Model file for the job. Use its own axes, mm. A direction names the side the tool comes from. Coordinates: 2 decimals unless noted, no trailing zeros. Loops run counter-clockwise (first coordinate to the right, second up) from the corner with the lowest first, then second, coordinate; pieces in that order, holes last.
from build123d import *

# Parameters (mm, degrees)
Y_KSEKLIK_EKSTR_ZYON1_DEPTH = 10
IZIM3_W                     = 33
IZIM3_H                     = 33
KES_EKSTR_ZYON1_DEPTH       = 10
KES_EKSTR_ZYON1_DRAFT       = -40.36453657
IZIM7_OUTSIDE_W             = 57.326
IZIM7_OUTSIDE_H             = 24.326
KES_EKSTR_ZYON6_DEPTH       = 56
IZIM10_OUTSIDE_W            = 24.326
IZIM10_OUTSIDE_H            = 57.326
KES_EKSTR_ZYON8_DEPTH       = 28
Y_KSEKLIK_EKSTR_ZYON2_DEPTH = 39
IZIM12_R                    = 14.5
Y_KSEKLIK_EKSTR_ZYON3_DEPTH = 100
Y_KSEKLIK_EKSTR_ZYON4_DEPTH = 2


with BuildPart() as part:
    # Çizim2 → Yükseklik-Ekstrüzyon1 (new body)
    with BuildSketch(Plane.XY):
        Polygon((0, 16.5), (0, 21.5), (-21.5, 21.5), (-21.5, 0), (-16.5, 0), (-16.5, 16.5), align=None)
        Polygon((0, 8), (0, 16.5), (-16.5, 16.5), (-16.5, 0), (-8, 0), (-8, 8), align=None)
        Polygon((-21.5, -21.5), (0, -21.5), (0, -16.5), (-16.5, -16.5), (-16.5, 0), (-21.5, 0), align=None)
        Polygon((-16.5, -16.5), (0, -16.5), (0, -8), (-8, -8), (-8, 0), (-16.5, 0), align=None)
        Polygon((21.5, -21.5), (21.5, 0), (16.5, 0), (16.5, -16.5), (0, -16.5), (0, -21.5), align=None)
        Polygon((16.5, -16.5), (16.5, 0), (8, 0), (8, -8), (0, -8), (0, -16.5), align=None)
        Polygon((8, 0), (16.5, 0), (16.5, 16.5), (0, 16.5), (0, 8), (8, 8), align=None)
        Polygon((16.5, 0), (21.5, 0), (21.5, 21.5), (0, 21.5), (0, 16.5), (16.5, 16.5), align=None)
    extrude(amount=Y_KSEKLIK_EKSTR_ZYON1_DEPTH)


with BuildPart() as kes_ekstr_zyon1_tool:
    # Çizim3 → Kes-Ekstrüzyon1 (with draft: the straight prism first)
    with BuildSketch(Plane.XY.offset(10)):
        Rectangle(IZIM3_W, IZIM3_H)
    extrude(amount=-KES_EKSTR_ZYON1_DEPTH)
    # Kes-Ekstrüzyon1: the draft: its side faces are tilted about the plane it starts from
    kes_ekstr_zyon1_sides = [kes_ekstr_zyon1_tool.faces().sort_by_distance(p)[0] for p in [
        (-16.5, 0, 5),
        (0, -16.5, 5),
        (16.5, 0, 5),
        (0, 16.5, 5),
    ]]
    draft(kes_ekstr_zyon1_sides, Plane.XY.offset(10), KES_EKSTR_ZYON1_DRAFT)


with BuildPart() as part_1:
    add(part.part)

    # Kes-Ekstrüzyon1: cut by kes_ekstr_zyon1_tool
    add(kes_ekstr_zyon1_tool.part, mode=Mode.SUBTRACT)

    # Çizim7 outside → Kes-Ekstrüzyon6 (cut)
    with BuildSketch(Plane(origin=(0, 21.5, 0), x_dir=(1, 0, 0), z_dir=(0, 1, 0))):
        with Locations((0, -5)):
            Rectangle(IZIM7_OUTSIDE_W, IZIM7_OUTSIDE_H)
        Polygon((-21.5, -10), (21.5, -10), (13, 0), (-13, 0), align=None, mode=Mode.SUBTRACT)
    extrude(amount=-KES_EKSTR_ZYON6_DEPTH, mode=Mode.SUBTRACT)

    # Çizim10 outside → Kes-Ekstrüzyon8 (cut, symmetric)
    with BuildSketch(Plane(origin=(0, 0, 0), x_dir=(0, 0, -1), z_dir=(1, 0, 0))):
        with Locations((-5, 0)):
            Rectangle(IZIM10_OUTSIDE_W, IZIM10_OUTSIDE_H)
        Polygon((-10, 21.5), (-10, -21.5), (0, -13), (0, 13), align=None, mode=Mode.SUBTRACT)
    extrude(amount=KES_EKSTR_ZYON8_DEPTH, both=True, mode=Mode.SUBTRACT)

    # Çizim11 → Yükseklik-Ekstrüzyon2 (add)
    with BuildSketch(Plane(origin=(0, 0, 0), x_dir=(-1, 0, 0), z_dir=(0, 0, -1))):
        Polygon((-13, -13), (-32.5, -32.5), (32.5, -32.5), (32.5, 32.5), (13, 13), (13, -13), align=None)
        Polygon((-32.5, 32.5), (-32.5, -32.5), (-13, -13), (-13, 13), (13, 13), (32.5, 32.5), align=None)
        Polygon((-13, 13), (-13, -13), (-8.000000001, -8.000000001), (-8, 8), (8.000000001, 8.000000001), (13, 13), align=None)
        Polygon((-8, 8), (-8.000000001, -8.000000001), (8.000000001, 8.000000001), align=None)
        Polygon((8.000000001, 8.000000001), (-8.000000001, -8.000000001), (8.000000001, -8.000000001), align=None)
        Polygon((-8.000000001, -8.000000001), (-13, -13), (13, -13), (13, 13), (8.000000001, 8.000000001), (8.000000001, -8.000000001), align=None)
    extrude(amount=Y_KSEKLIK_EKSTR_ZYON2_DEPTH)

    # Çizim12 → Yükseklik-Ekstrüzyon3 (add)
    with BuildSketch(Plane.XZ.offset(32.5)):
        with Locations((0, -19.5)):
            Circle(IZIM12_R)
    extrude(amount=Y_KSEKLIK_EKSTR_ZYON3_DEPTH)

    # Çizim13 → Yükseklik-Ekstrüzyon4 (add)
    with BuildSketch(Plane.XZ.offset(132.5)):
        Polygon((-1, -31.880933569), (1, -31.880933569), (0, -33.652876783), align=None)
        Polygon((-3.663034054, -33.170629201), (-2.238495577, -31.717882533), (-4.17034723, -31.200244443), align=None)
        Polygon((-7.076438392, -31.756750831), (-5.324441381, -30.722202993), (-7.056492188, -29.722202993), align=None)
        Polygon((-10.007595147, -29.507595147), (-8.047535303, -28.961748865), (-9.461748865, -27.547535303), align=None)
        Polygon((-12.256750831, -26.576438392), (-10.222202993, -26.556492188), (-11.222202993, -24.824441381), align=None)
        Polygon((-13.670629201, -23.163034054), (-11.700244443, -23.67034723), (-12.217882533, -21.738495578), align=None)
        Polygon((-14.152876783, -19.5), (-12.380933569, -20.5), (-12.380933569, -18.5), align=None)
    extrude(amount=Y_KSEKLIK_EKSTR_ZYON4_DEPTH)


solid = part_1.part
Q1. Which spindle directions (+Z, -Z, +X, -X, +Y, -Y) get a long thin tool onto all of the face, cutting with end or side? Do faces 4 (the flat face through (17.31, 0.3, 5.07)), 5 (the flat face through (-13.254, -0.231, 6.181)), 6 (the flat face through (0.3, 17.19, 4.93)). Say none if no direction does.
Answers:
face 4: +X, +Y, -Y
face 5: +Z
face 6: +X, -X, +Y
Q2. Drill centre lines: line 1 (Z direction, x = -3, y = -49.5); line 2 (Y direction, x = -9.5, z = -22.5); line 3 (Y direction, x = 10, z = -8). Where is each one in solid material? Low to high.
Answers:
line 1: z = -33.69 to -5.31
line 2: y = -132.5 to 32.5
line 3: y = -32.5 to 32.5
Q3. Mould opens along Y. For faces 1 (the flat face through (0, 0, 0)), 2 (the flat face through (0, 0, -39)), 3 (the flat face through (0, 32.5, -19)) say: +Y half, -Y half, draft (parallel to the pull), parting line (faces both ways), or undercut.
Answers:
face 1: undercut
face 2: draft
face 3: +Y half
Q4. Slice it at B-B (z = -9). List the corners of the cut face in (x, y), and give its area (4 significant figures).
Answers:
outline: (-32.5, -32.5) - (-10, -32.5) - (-10, -132.5) - (10, -132.5) - (10, -32.5) - (32.5, -32.5) - (32.5, 32.5) - (-32.5, 32.5) - close
area: 6,225 mm2
Q5. Slice it at C-C (z = 4.5). List the corners of the cut face in (x, y) (3 decimals).
Answers:
outline: (-16.825, -16.825) - (16.825, -16.825) - (16.825, 16.825) - (-16.825, 16.825) - close; hole (-11.825, -11.825) - (11.825, -11.825) - (11.825, 11.825) - (-11.825, 11.825) - close
Q6. Flat gauge pins, fed straight in: P1, Ø4, axis at x = 3, z = -3, coming from the -Y side; P2, Ø1.5, axis at y = -96.5, z = -10.5, coming from the -X side; P3, Ø11.5, axis at x = -5, z = -16.5, coming from the -Y side. Where does each tip first touch, or does it go through?
Answers:
P1: stops at y = -32.5
P2: stops at x = -11.92
P3: stops at y = -132.5
Q7. Slice it at D-D (y = -72). List the corners of the cut face in (x, z), and give its area (3 significant figures).
Answers:
outline: circle Ø29 at (0, -19.5)
area: 661 mm2
Q8. Slice it at A-A (y = 20). List the corners of the cut face in (x, z), and give its area (3 significant figures).
Answers:
outline: (-32.5, -39) - (32.5, -39) - (32.5, 0) - (-32.5, 0) - close; (-21.5, 10) - (-20, 8.24) - (20, 8.24) - (21.5, 10) - close
area: 2,610 mm2
